Source: CAD feature listing. Evaluate the final solid. Frame: model axes, mm. Face numbers are marked on the shaded views. A direction names the side the tool comes from. Round coordinates to 2 decimals unless told otherwise and drop trailing zeros. Write each loop counter-clockwise with the first axis right and the second up, starting at its lowest first coordinate (ties: lowest second). Pieces come first, ordered by that corner, then holes. Notation, with made-up numbers: (58, 46.25) -> (88, 46.25) arc R10 cw to (88, 58.25) -> close; hole circle Ø2 at (73.25, 86.25). An arc over 180 degrees is marked (long way). Put each result on its own line as item: value.
```python
from build123d import *

# Parameters (mm, degrees)
BOSS_EXTRUDE1_DEPTH       = 8.13
F_3_0MM_DOWEL_HOLE1_D     = 3
F_3_0MM_DOWEL_HOLE1_DEPTH = 35
F_3_0MM_DOWEL_HOLE1_TIP   = 0.901290929


with BuildPart() as part:
    # Sketch1 → Boss-Extrude1 (new body)
    with BuildSketch(Plane.XY):
        with BuildLine():
            Line((-9.035, 0), (-9.035, 2))
            Line((-9.035, 2), (-4.035, 2))
            Line((-4.035, 2), (-4.035, 1.53))
            ThreePointArc((-4.035, 1.53), (-4.005710678, 1.459289322), (-3.935, 1.43))
            Line((-3.935, 1.43), (3.935, 1.43))
            ThreePointArc((3.935, 1.43), (4.005710678, 1.459289322), (4.035, 1.53))
            Line((4.035, 1.53), (4.035, 2))
            Line((4.035, 2), (9.035, 2))
            Line((9.035, 2), (9.035, 0))
            Line((9.035, 0), (-9.035, 0))
        make_face()
    extrude(amount=BOSS_EXTRUDE1_DEPTH)

    # Ø3.0mm Dowel Hole1
    with Locations(Plane(origin=(0, 2, 0), x_dir=(1, 0, 0), z_dir=(0, 1, 0))):
        with Locations((6.335, -4.08), (-6.335, -4.08)):
            Hole(F_3_0MM_DOWEL_HOLE1_D / 2, depth=F_3_0MM_DOWEL_HOLE1_DEPTH)
            with Locations((0, 0, -(F_3_0MM_DOWEL_HOLE1_DEPTH + F_3_0MM_DOWEL_HOLE1_TIP / 2))):  # 118° drill point
                Cone(0, F_3_0MM_DOWEL_HOLE1_D / 2, F_3_0MM_DOWEL_HOLE1_TIP, mode=Mode.SUBTRACT)


solid = part.part
```
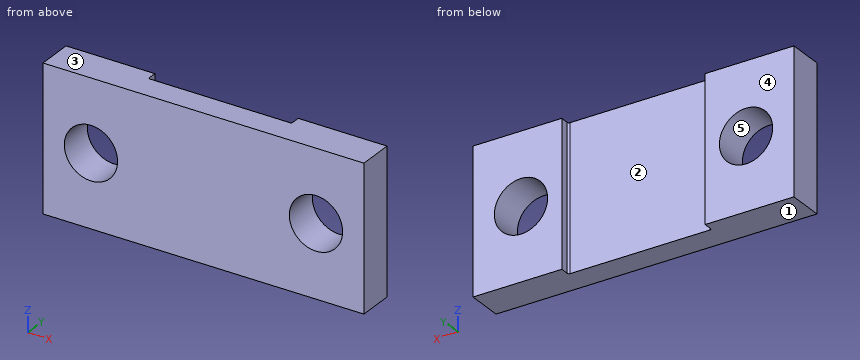
Q1. Cut plane D-D on z = 1.5. Output: boundary loops of the cut face in (x, y) (3 decimals).
Ans:
outline: (-9.035, 0) -> (9.035, 0) -> (9.035, 2) -> (4.035, 2) -> (4.035, 1.53) arc R0.1 cw to (3.935, 1.43) -> (-3.935, 1.43) arc R0.1 cw to (-4.035, 1.53) -> (-4.035, 2) -> (-9.035, 2) -> close
Q2. Material intervals for line 1 (X direction, y = 1.2, z = 4.08) (3 decimals); line 2 (Z direction, x = -6.25, y = 1.85); line 3 (X direction, y = 1.1, z = 3) (3 decimals), sorted ascending. Write a range as [from, to].
Ans:
line 1: x = [-9.035, -7.835], [-4.835, 4.835], [7.835, 9.035]
line 2: z = [0, 2.58], [5.58, 8.13]
line 3: x = [-9.035, -7.376], [-5.294, 5.294], [7.376, 9.035]
Q3. Draft query along Z for the marked faces 3, 4 and 5. Return one class per face: +Z half, -Z half, draft (parallel to the pull), parting line (faces both ways), or undercut.
Ans:
face 3: +Z half
face 4: draft
face 5: undercut
Q4. Cut plane B-B on z = 4.08. Output: boundary loops of the cut face in (x, y) (3 decimals), and give its area (3 significant figures).
Ans:
outline: (-9.035, 0) -> (-7.835, 0) -> (-7.835, 2) -> (-9.035, 2) -> close; (-4.835, 0) -> (4.835, 0) -> (4.835, 2) -> (4.035, 2) -> (4.035, 1.53) arc R0.1 cw to (3.935, 1.43) -> (-3.935, 1.43) arc R0.1 cw to (-4.035, 1.53) -> (-4.035, 2) -> (-4.835, 2) -> close; (7.835, 0) -> (9.035, 0) -> (9.035, 2) -> (7.835, 2) -> close
area: 19.5 mm^2
Q5. Reachability of the marked faces 1 and 2 from +Z, -Z, +X, -X, +Y, -Y: full face, straight path, thin tool, end or side. Return the list, or none.
Ans:
face 1: -Z, +X, -X, +Y, -Y
face 2: +Z, -Z, +Y
Q6. Pin query (flat end, axial travel): pin 1 (1.5 mm diameter, centred on x = -4, z = 1, fed in from +Y); pin 2 (2.5 mm diameter, centred on x = -6.335, z = 4.08, fed in from -Y). Return the tip coordinate at first contact, or that it passes through.
Ans:
pin 1: stops at y = 2
pin 2: passes through
Q7. Cut plane A-A on y = 1.8. Output: boundary loops of the cut face in (x, z) (3 decimals).
Ans:
outline: (-9.035, 0) -> (-4.035, 0) -> (-4.035, 8.13) -> (-9.035, 8.13) -> close; (4.035, 0) -> (9.035, 0) -> (9.035, 8.13) -> (4.035, 8.13) -> close; hole circle Ø3 at (-6.335, 4.08); hole circle Ø3 at (6.335, 4.08)
Q8. Cut plane C-C on y = 0.3. Output: boundary loops of the cut face in (x, z) (3 decimals), and give its area (3 significant figures).
Ans:
outline: (-9.035, 0) -> (9.035, 0) -> (9.035, 8.13) -> (-9.035, 8.13) -> close; hole circle Ø3 at (-6.335, 4.08); hole circle Ø3 at (6.335, 4.08)
area: 133 mm^2
